```python
from build123d import *

# Parameters (mm, degrees)
F0_W     = 40
F0_H     = 40
F1_DEPTH = 5


with BuildPart() as f1:
    # F0 (on Top) → F1 (new body)
    with BuildSketch(Plane.XY):
        Rectangle(F0_W, F0_H)
    extrude(amount=F1_DEPTH)

    # F2 (on Front) → F3 (revolve)
    with BuildSketch(Plane.XZ):
        Polygon((-14, 26.329274), (-14, 5), (-11.5, 5), (-11.5, 25), align=None)
    revolve(axis=Axis((0, 0, 17.722977), (0, 0, -1)))


solid = f1.part
```
The listing builds one solid part. Answer for the finished solid, in the listing's coordinates (mm). A direction names the side the tool comes from. Coordinates: 2 decimals unless noted, no trailing zeros. Write each loop counter-clockwise with the first axis right and the second up, starting at its lowest first coordinate (ties: lowest second). Pieces come first, ordered by that corner, then holes. Notation, with made-up numbers: M 49.25,80 L 106.25,80 A17 cw 106.25,85 Z; hole C 31,30 d1. An arc over 180 degrees is marked long. Use a Markdown table: item, result. Add a question column.
1. Section B-B (z = 22.25) is taken. Give the vertices of the cut face in (x, y), plus the area to 3 significant figures.
2. Which of the six approach directions +Z, -Z, +X, -X, +Y, -Y give full straight-line access (tool end or side, diameter ignored) to faces 1 (the cylindrical face through (-12.932, -5.362, 15.515)), 2 (the flat face through (-20, 0, 2))?
3. For a pull along Y with two mould halves and no side action, classify faces 3 (the conical face through (2.527, -11.379, 25.083)), 4 (the flat face through (20, 0, 2)), 5 (the flat face through (0, 20, 2)) as +Y half, -Y half, draft (parallel to the pull), parting line (faces both ways), or undercut.
4. Straight lines are drawn through the part: line 1 along Y through (x, z) = (0, 13.75); line 2 along Z through (x, y) = (6.5, 1); line 3 along Y through (x, z) = (-2, 13). For each, find the intervals that lie inside material, in ascending order. Write a range as [from, to].
5. Given P1, Ø12, axis at y = 15.5, z = 13.5, coming from the +X side; P2, Ø4, axis at y = 4, z = 22, coming from the -X side; P3, Ø8, axis at x = -7.5, z = 18.5, coming from the +Y side, each flat-ended and moving along its own axis, determine where each tip first touches the part or whether it passes through.
6. Section A-A (x = 0) is taken. Give the vertices of the cut face in (y, z), plus the area to 3 significant figures.
Data:
| question | item | result |
|---|---|---|
| 1 | outline | C 0,0 d28; hole C 0,0 d23 |
| 1 | area | 200 mm2 |
| 2 | face 1 | +Z |
| 2 | face 2 | +Z, -Z, -X, +Y, -Y |
| 3 | face 3 | undercut |
| 3 | face 4 | draft |
| 3 | face 5 | +Y half |
| 4 | line 1 | y = [-14, -11.5], [11.5, 14] |
| 4 | line 2 | z = [0, 5] |
| 4 | line 3 | y = [-13.86, -11.32], [11.32, 13.86] |
| 5 | P1 | stops at x = 10.28 |
| 5 | P2 | stops at x = -13.86 |
| 5 | P3 | stops at y = 13.56 |
| 6 | outline | M -20,0 L 20,0 L 20,5 L 14,5 L 14,26.33 L 11.5,25 L 11.5,5 L -11.5,5 L -11.5,25 L -14,26.33 L -14,5 L -20,5 Z |
| 6 | area | 303 mm2 |
